```python
from build123d import *

# Parameters (mm, degrees)
F2_R     = 11.43
F2_R_2   = 1.5875
F3_DEPTH = 1.27
F5_R     = 11.43
F5_R_2   = 1.5875
F6_DEPTH = 1.27


# Not quite as in the source:
# - a variable given as a bare number and used for a length is read in inches; the dataset says mm whatever the document's units were


with BuildPart() as f3:
    # F2 (on offset) → F3 (new body)
    with BuildSketch(Plane.XZ.offset(11.43)):
        Circle(F2_R)
        Circle(F2_R_2, mode=Mode.SUBTRACT)
    extrude(amount=F3_DEPTH)



with BuildPart() as f6:
    # F5 (on offset) → F6 (new body)
    with BuildSketch(Plane.XZ.offset(-11.43)):
        Circle(F5_R)
        Circle(F5_R_2, mode=Mode.SUBTRACT)
    extrude(amount=-F6_DEPTH)


with BuildPart() as f3_1:
    add(f3.part)

    add(f6.part)  # F8 merges F6
    # F7 (on Right) → F8 (revolve)
    with BuildSketch(Plane.YZ):
        with BuildLine():
            ThreePointArc((11.43, 11.43), (0, 7.8646021863), (-11.43, 11.43))
            Line((-11.43, 11.43), (-11.43, 1.5875))
            Line((-11.43, 1.5875), (11.43, 1.5875))
            Line((11.43, 1.5875), (11.43, 11.43))
        make_face()
    revolve(axis=Axis((0, 0, 0), (0, -1, 0)))


solid = f3_1.part
```
Can you work these out from the model? Positions are in its coordinate system, mm. Round coordinates to 2 decimals unless told otherwise and drop trailing zeros. Loops run counter-clockwise (first coordinate to the right, second up) from the corner with the lowest first, then second, coordinate; pieces in that order, holes last. Notation, with made-up numbers: M 54,88.25 L 62,88.25 A22 cw 62,117.25 Z; hole C 6,-22 d4. An arc over 180 degrees is marked long. Answer in a Markdown table with one row per item.
1. If we section it at B-B, the plane z = 0: Please give me the cut outline in (x, y).
Established:
| item | result |
|---|---|
| outline | M -11.43,-12.7 L -1.59,-12.7 L -1.59,12.7 L -11.43,12.7 L -11.43,11.43 A20.1 cw -11.43,-11.43 Z; M 1.59,-12.7 L 11.43,-12.7 L 11.43,-11.43 A20.1 cw 11.43,11.43 L 11.43,12.7 L 1.59,12.7 Z |
2. I'm going to push flat-ended pins straight in: pin 1 Ø8 at (x, y) = (3, 0.5) entering from +Z; pin 2 Ø2 at (x, y) = (8.5, -9.5) entering from +Z; pin 3 Ø10 at (x, y) = (7, 1) entering from +Z. Where does each tip first touch, or does it pass through?
Established:
| item | result |
|---|---|
| pin 1 | z = 8.2 |
| pin 2 | z = 7.26 |
| pin 3 | z = 7.72 |
3. If we section it at A-A, the plane x = 0: Please give me the cut outline in (y, z), plus the area to 3 significant figures.
Established:
| item | result |
|---|---|
| outline | M -12.7,-11.43 L -11.43,-11.43 A20.1 cw 11.43,-11.43 L 12.7,-11.43 L 12.7,-1.59 L -12.7,-1.59 Z; M -12.7,1.59 L 12.7,1.59 L 12.7,11.43 L 11.43,11.43 A20.1 cw -11.43,11.43 L -12.7,11.43 Z |
| area | 389 mm² |
4. If we section it at D-D, the plane y = 2.5: Please give me the cut outline in (x, z) (1 decimal).
Established:
| item | result |
|---|---|
| outline | C 0,0 d16; hole C 0,0 d3.2 |
5. Please list where these lines run through material, in increasing order: line 1 (Z direction, x = 0, y = -11.8); line 2 (X direction, y = -3.5, z = 1). Write a range as from..to.
Established:
| item | result |
|---|---|
| line 1 | -11.43..-1.59, 1.59..11.43 |
| line 2 | -8.11..-1.23, 1.23..8.11 |
6. If we section it at C-C, the plane y = 7.75: Please give me the cut outline in (x, z) (1 decimal).
Established:
| item | result |
|---|---|
| outline | C 0,0 d18.8; hole C 0,0 d3.2 |
